Could you check a few things on this model? Use its own coordinates, in mm. Give positions to 0.01 mm unless a question says otherwise; leave off trailing zeros. Order: outer loops, then holes, each group sorted by start corner. A loop starts at its lowest first (then second) coordinate and runs counter-clockwise, first axis right, second up. Notation, with made-up numbers: M -20,-2.5 L 13,-2.5 A18 ccw 13,26.5 Z; hole C 59,68.5 d9. An arc over 180 degrees is marked long. Use a Markdown table: item, result. Add a question column.
Item 1: Suppose I cut it at B-B on z = 10.5. Count the separate pieces of the cut face and the enclosed holes in it, plus the area to 3 significant figures.
Item 2: If I drill on L1, parallel to X at y = 0, z = 11; L2, parallel to Y at x = -18.5, z = 2.5; L3, parallel to X at y = -44.5, z = 9.5, over which ranges is the centre line in solid material (lowest first)? Write a range as from..to.
Item 3: Suppose I cut it at A-A on y = 0. Write out the boundary of the cut face in (x, z).
Item 4: I'm going to push flat-ended pins straight in: pin 1 Ø5.5 at (x, y) = (31.75, -47.5) entering from +Z; pin 2 Ø3 at (x, y) = (79.25, 0) entering from -Z; pin 3 Ø6 at (y, z) = (25, 10) entering from +X; pin 4 Ø1.5 at (x, z) = (44.5, 3) entering from +Y. Where does each tip first touch, or does it pass through?
Item 5: Suppose I cut it at D-D on y = 31.5. Write out the boundary of the cut face in (x, z), plus the area to 3 significant figures.
Item 6: Suppose I cut it at C-C on y = 47.5. Write out the boundary of the cut face in (x, z), plus the area to 3 significant figures.
from build123d import *

# Parameters (mm, degrees)
RESSALTO_EXTRUS_O4_DEPTH = 12.5
CORTE_EXTRUS_O2_DEPTH    = 6.25
FURO5_D                  = 5
FURO5_CBORE_D            = 9
FURO5_CBORE_DEPTH        = 5
PADR_OCIRCULAR3_COUNT    = 7
PADR_OCIRCULAR3_ANGLE    = 180
FURO6_D                  = 5
FURO6_CBORE_D            = 9
FURO6_CBORE_DEPTH        = 5
PADR_OCIRCULAR4_COUNT    = 7
PADR_OCIRCULAR4_ANGLE    = 180


with BuildPart() as part:
    # Esbo_o1 → Ressalto-extrus_o4 (new body)
    # profile 1 of 2: a face of its own
    with BuildSketch(Plane.XY):
        with BuildLine():
            Line((-31.75, -61), (31.75, -61))
            ThreePointArc((31.75, -61), (92.75, 0), (31.75, 61))
            Line((31.75, 61), (-31.75, 61))
            ThreePointArc((-31.75, 61), (-92.75, 0), (-31.75, -61))
        make_face()
        with BuildLine():
            ThreePointArc((31.75, -11.5), (43.25, 0), (31.75, 11.5))
            Line((31.75, 11.5), (-31.75, 11.5))
            ThreePointArc((-31.75, 11.5), (-43.25, 0), (-31.75, -11.5))
            Line((-31.75, -11.5), (31.75, -11.5))
        make_face(mode=Mode.SUBTRACT)
    # profile 2 of 2: a face of its own
    with BuildSketch(Plane.XY):
        with BuildLine():
            Line((-31.75, -11.5), (31.75, -11.5))
            ThreePointArc((31.75, -11.5), (43.25, 0), (31.75, 11.5))
            Line((31.75, 11.5), (-31.75, 11.5))
            ThreePointArc((-31.75, 11.5), (-43.25, 0), (-31.75, -11.5))
        make_face()
    extrude(amount=RESSALTO_EXTRUS_O4_DEPTH)

    # Esbo_o1_7 → Corte-extrus_o2 (cut)
    with BuildSketch(Plane.XY):
        with BuildLine():
            Line((-31.75, -11.5), (31.75, -11.5))
            ThreePointArc((31.75, -11.5), (43.25, 0), (31.75, 11.5))
            Line((31.75, 11.5), (-31.75, 11.5))
            ThreePointArc((-31.75, 11.5), (-43.25, 0), (-31.75, -11.5))
        make_face()
    extrude(amount=CORTE_EXTRUS_O2_DEPTH, mode=Mode.SUBTRACT)

    # Furo5 (through all)
    with Locations(Plane.XY.offset(12.5)):
        with Locations((-31.75, 47.5)):
            furo5 = CounterBoreHole(FURO5_D / 2, FURO5_CBORE_D / 2, FURO5_CBORE_DEPTH)

    # Padr_oCircular3: Furo5 ×7 about axis
    padr_ocircular3_axis = Axis((-31.75, 0, 0), (0, 0, 1))
    for i in range(1, PADR_OCIRCULAR3_COUNT):
        add(furo5.rotate(padr_ocircular3_axis, i * PADR_OCIRCULAR3_ANGLE / (PADR_OCIRCULAR3_COUNT - 1)), mode=Mode.SUBTRACT)

    # Furo6 (through all)
    with Locations(Plane.XY.offset(12.5)):
        with Locations((31.75, 47.5)):
            furo6 = CounterBoreHole(FURO6_D / 2, FURO6_CBORE_D / 2, FURO6_CBORE_DEPTH)

    # Padr_oCircular4: Furo6 ×7 about axis
    padr_ocircular4_axis = Axis((31.75, 0, 0), (0, 0, -1))
    for i in range(1, PADR_OCIRCULAR4_COUNT):
        add(furo6.rotate(padr_ocircular4_axis, i * PADR_OCIRCULAR4_ANGLE / (PADR_OCIRCULAR4_COUNT - 1)), mode=Mode.SUBTRACT)


solid = part.part
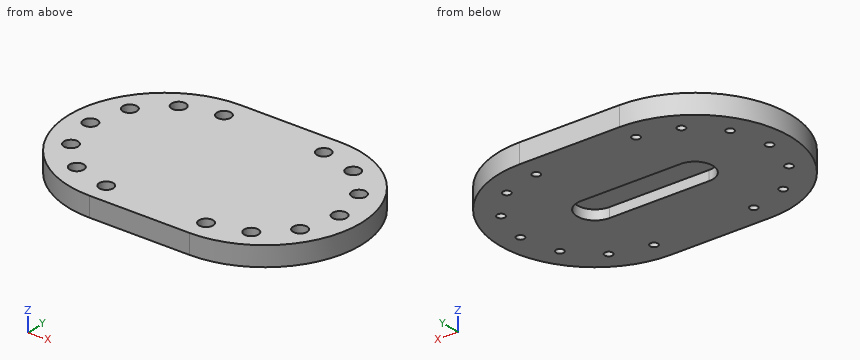
Findings below:
| question | item | result |
|---|---|---|
| 1 | separate pieces | 1 |
| 1 | enclosed holes | 14 |
| 1 | area | 18,500 mm^2 |
| 2 | L1 | x = -92.75..-83.75, -74.75..74.75, 83.75..92.75 |
| 2 | L2 | y = -61..-11.5, 11.5..61 |
| 2 | L3 | x = -73.47..-58.49, -52.51..-35.1, -28.4..28.4, 35.1..52.51, 58.49..73.47 |
| 3 | outline | M -92.75,0 L -81.75,0 L -81.75,7.5 L -83.75,7.5 L -83.75,12.5 L -92.75,12.5 Z; M -76.75,0 L -43.25,0 L -43.25,6.25 L 43.25,6.25 L 43.25,0 L 76.75,0 L 76.75,7.5 L 74.75,7.5 L 74.75,12.5 L -74.75,12.5 L -74.75,7.5 L -76.75,7.5 Z; M 81.75,0 L 92.75,0 L 92.75,12.5 L 83.75,12.5 L 83.75,7.5 L 81.75,7.5 Z |
| 4 | pin 1 | stops at z = 7.5 |
| 4 | pin 2 | passes through |
| 4 | pin 3 | stops at x = 88.64 |
| 4 | pin 4 | stops at y = 59.81 |
| 5 | outline | M -83.99,0 L 83.99,0 L 83.99,12.5 L -83.99,12.5 Z |
| 5 | area | 2,100 mm^2 |
| 6 | outline | M -70.02,0 L -34.25,0 L -34.25,7.5 L -36.25,7.5 L -36.25,12.5 L -70.02,12.5 Z; M -29.25,0 L 29.25,0 L 29.25,7.5 L 27.25,7.5 L 27.25,12.5 L -27.25,12.5 L -27.25,7.5 L -29.25,7.5 Z; M 34.25,0 L 70.02,0 L 70.02,12.5 L 36.25,12.5 L 36.25,7.5 L 34.25,7.5 Z |
| 6 | area | 1,590 mm^2 |
